Build history of the part. All positions in model axes, mm. A direction names the side the tool comes from. Coordinates: 2 decimals unless noted, no trailing zeros. Loops run counter-clockwise (first coordinate to the right, second up) from the corner with the lowest first, then second, coordinate; pieces in that order, holes last.
Item 1: Cut at D-D (x = 4). List the corners of the cut face in (y, z), and give its area (3 significant figures).
Item 2: 3-axis set-ups, long thin cutter, end or side, ignore diameter. For faces 1 (the face through (0, -4.5, -1)), 2 (the face through (-2.4, -10.2, 18)), 3 (the face through (-13, -2, 0)): which of +Z, -Z, +X, -X, +Y, -Y reach the whole face in a straight line?
Item 3: Drill centre lines: line 1 along Y through (x, z) = (-5, 18); line 2 along Y through (x, z) = (2, 3); line 3 along X through (y, z) = (-9.5, 20.5). Where is each one in solid material? Low to high.
Item 4: Cut at C-C (z = -7). List the corners of the cut face in (x, y).
Item 5: Mould opens along X. For faces 4 (the face through (8.5, -7, 18)), 5 (the face through (-5.51, -13.5, 18.07)), 6 (the face through (10.9, -2.3, -8.2)) say: released by +X, released by -X, zero draft, split by the parting line, or undercut.
Item 6: Cut at A-A (x = 12.5). List the corners of the cut face in (y, z).
Item 7: Cut at B-B (y = -12). List the corners of the cut face in (x, z), and give its area (3 significant figures).
Item 8: Flat gauge pins, fed straight in: pin 1 (2.5 mm diameter, centred on y = -12, z = 18, fed in from +X); pin 2 (21 mm diameter, centred on x = -7.5, z = 4, fed in from -Y); pin 3 (10 mm diameter, centred on x = -3, z = 5, fed in from +Y); pin 4 (3 mm diameter, centred on x = -0.5, y = -11.5, fed in from -Z). Where does each tip first touch, or does it go through?
from build123d import *

# Parameters (mm, degrees)
F0_W      = 35
F0_H      = 45
F1_DEPTH  = 4.5
F2_R      = 2
F3_DEPTH  = 10
F4_W      = 35
F4_H      = 10
F5_DEPTH  = 12.5
F6_R      = 3
F7_DEPTH  = 6
F8_W      = 35
F8_H      = 4.5
F9_DEPTH  = 2
F10_W     = 9
F10_H     = 25
F11_DEPTH = 17.001
F12_R     = 1.5
F13_DEPTH = 26.001
F14_W     = 35
F14_H     = 6
F15_DEPTH = 4.501
F16_W     = 35
F16_H     = 4.5
F17_DEPTH = 1


with BuildPart() as f1:
    # F0 (on Front) → F1 (new body)
    with BuildSketch(Plane.XZ):
        with Locations((0, 2.5)):
            Rectangle(F0_W, F0_H)
    extrude(amount=F1_DEPTH)

    # F2 (on face) → F3 (cut)
    with BuildSketch(Plane.XZ.offset(4.5)):
        with Locations((12.5, -15)):
            Circle(F2_R)
        with Locations((-12.5, -15)):
            Circle(F2_R)
        with Locations((-12.5, -7)):
            Circle(F2_R)
        with Locations((12.5, -7)):
            Circle(F2_R)
    extrude(amount=-F3_DEPTH, mode=Mode.SUBTRACT)

    # F4 (on face) → F5 (join)
    with BuildSketch(Plane.XZ.offset(4.5)):
        with Locations((0, 20)):
            Rectangle(F4_W, F4_H)
    extrude(amount=F5_DEPTH)

    # F6 (on face) → F7 (cut)
    with BuildSketch(Plane(origin=(0, 0, 15), x_dir=(1, 0, 0), z_dir=(0, 0, -1))):
        with Locations((0, 12)):
            Circle(F6_R)
    extrude(amount=-F7_DEPTH, mode=Mode.SUBTRACT)

    # F8 (on face) → F9 (cut)
    with BuildSketch(Plane(origin=(0, 0, -20), x_dir=(1, 0, 0), z_dir=(0, 0, -1))):
        with Locations((0, 2.25)):
            Rectangle(F8_W, F8_H)
    extrude(amount=-F9_DEPTH, mode=Mode.SUBTRACT)

    # F10 (on face) → F11 (cut, through all)
    with BuildSketch(Plane.XZ.offset(17)):
        with Locations((-13, 12.5)):
            Rectangle(F10_W, F10_H)
        with Locations((13, 12.5)):
            Rectangle(F10_W, F10_H)
    extrude(amount=-F11_DEPTH, mode=Mode.SUBTRACT)

    # F12 (on face) → F13 (cut, through all)
    with BuildSketch(Plane.YZ.offset(8.5)):
        with Locations((-12, 18)):
            Circle(F12_R)
    extrude(amount=-F13_DEPTH, mode=Mode.SUBTRACT)

    # F14 (on face) → F15 (cut, through all)
    with BuildSketch(Plane.XZ.offset(4.5)):
        with Locations((0, -15)):
            Rectangle(F14_W, F14_H)
    extrude(amount=-F15_DEPTH, mode=Mode.SUBTRACT)

    # F16 (on face) → F17 (cut)
    with BuildSketch(Plane(origin=(0, 0, -12), x_dir=(1, 0, 0), z_dir=(0, 0, -1))):
        with Locations((0, 2.25)):
            Rectangle(F16_W, F16_H)
    extrude(amount=-F17_DEPTH, mode=Mode.SUBTRACT)


solid = f1.part
Filled sheet:
1. outline: (-17, 15) - (-4.5, 15) - (-4.5, -11) - (0, -11) - (0, 25) - (-17, 25) - close; hole circle Ø3 at (-12, 18)
1. area: 280 mm2
2. face 1: -Z, +X, -X, -Y
2. face 2: -Z
2. face 3: +Z, -X, +Y, -Y
3. line 1: y = -17 to -13.5, -10.5 to 0
3. line 2: y = -4.5 to 0
3. line 3: x = -8.5 to -1.66, 1.66 to 8.5
4. outline: (-17.5, -4.5) - (-14.5, -4.5) - (-14.5, 0) - (-17.5, 0) - close; (-10.5, -4.5) - (10.5, -4.5) - (10.5, 0) - (-10.5, 0) - close; (14.5, -4.5) - (17.5, -4.5) - (17.5, 0) - (14.5, 0) - close
5. face 4: released by +X
5. face 5: zero draft
5. face 6: undercut
6. outline: (-4.5, -11) - (0, -11) - (0, -9) - (-4.5, -9) - close; (-4.5, -5) - (0, -5) - (0, 0) - (-4.5, 0) - close
7. outline: (-8.5, 15) - (-3, 15) - (-3, 16.5) - (-8.5, 16.5) - close; (-8.5, 19.5) - (-3, 19.5) - (-3, 21) - (3, 21) - (3, 19.5) - (8.5, 19.5) - (8.5, 25) - (-8.5, 25) - close; (3, 15) - (8.5, 15) - (8.5, 16.5) - (3, 16.5) - close
7. area: 101 mm2
8. pin 1: passes through
8. pin 2: stops at y = -4.5
8. pin 3: stops at y = 0
8. pin 4: stops at z = 21
